Source: CAD feature listing. Evaluate the final solid. Frame: model axes, mm. Give positions to 0.01 mm unless a question says otherwise; leave off trailing zeros. Order: outer loops, then holes, each group sorted by start corner. A loop starts at its lowest first (then second) coordinate and runs counter-clockwise, first axis right, second up.
from build123d import *

# Parameters (mm, degrees)
BOSS_EXTRUDE1_DEPTH = 25
SKETCH3_R           = 1.25
CUT_EXTRUDE1_DEPTH  = 20


with BuildPart() as part:
    # Sketch2 → Boss-Extrude1 (new body)
    with BuildSketch(Plane(origin=(0, 0, 0), x_dir=(1, 0, 0), z_dir=(0, 1, 0))):
        with BuildLine():
            Line((0, -33.8431677), (-12.5, -33.8431677))
            Line((-12.5, -33.8431677), (-12.5, -35.991110013))
            ThreePointArc((-12.5, -35.991110013), (0, -38.1), (12.5, -35.991110013))
            Line((12.5, -35.991110013), (12.5, -33.8431677))
            Line((12.5, -33.8431677), (0, -33.8431677))
        make_face()
    extrude(amount=BOSS_EXTRUDE1_DEPTH)

    # Sketch3 → Cut-Extrude1 (cut)
    with BuildSketch(Plane(origin=(0, 0, 33.8431677), x_dir=(-1, 0, 0), z_dir=(0, 0, -1))):
        with Locations((0, 12.5)):
            Circle(SKETCH3_R)
    extrude(amount=-CUT_EXTRUDE1_DEPTH, mode=Mode.SUBTRACT)


solid = part.part
1) Section query C-C on z = 36.55. Output: boundary loops of the cut face in (x, y), and give its area (3 significant figures).
Checks:
outline: (-10.76, 0) - (10.76, 0) - (10.76, 25) - (-10.76, 25) - close; hole circle Ø2.5 at (0, 12.5)
area: 533 mm2
2) Section query B-B on y = 12.5. Output: boundary loops of the cut face in (x, z), and give its area (3 significant figures).
Checks:
outline: (-12.5, 33.84) - (-1.25, 33.84) - (-1.25, 38.08) arc R38.1 ccw to (-12.5, 35.99) - close; (1.25, 33.84) - (12.5, 33.84) - (12.5, 35.99) arc R38.1 ccw to (1.25, 38.08) - close
area: 78.4 mm2
3) Pull-direction query (Y, two-part tool) for faces 1 (the face through (0, 0, 35)), 2 (the face through (0, 25, 35)), 3 (the face through (12.5, 12, 35)), 4 (the face through (0.16, 13.74, 35.94)); classes: +Y half, -Y half, draft (parallel to the pull), parting line (faces both ways), or undercut.
Checks:
face 1: -Y half
face 2: +Y half
face 3: draft
face 4: undercut
4) First-contact query: pin 1 Ø1 at (x, y) = (5, 13) entering from +Z. Flat tip, straight axial feed; report the tip coordinate or a pass-through.
Checks:
pin 1: stops at z = 37.83
5) Section query A-A on x = 0. Output: boundary loops of the cut face in (y, z).
Checks:
outline: (0, 33.84) - (11.25, 33.84) - (11.25, 38.1) - (0, 38.1) - close; (13.75, 33.84) - (25, 33.84) - (25, 38.1) - (13.75, 38.1) - close
6) Ray query, L1, parallel to X at y = 12.5, z = 35.55; L2, parallel to Y at x = 0, z = 37.05; L3, parallel to Z at x = 0.5, y = 10.5. Return the intervals inside material, ascending.
Checks:
L1: x = -12.5 to -1.25, 1.25 to 12.5
L2: y = 0 to 11.25, 13.75 to 25
L3: z = 33.84 to 38.1
7) Section query D-D on y = 3.75. Output: boundary loops of the cut face in (x, z), and give its area (3 significant figures).
Checks:
outline: (-12.5, 33.84) - (12.5, 33.84) - (12.5, 35.99) arc R38.1 ccw to (-12.5, 35.99) - close
area: 89.0 mm2
